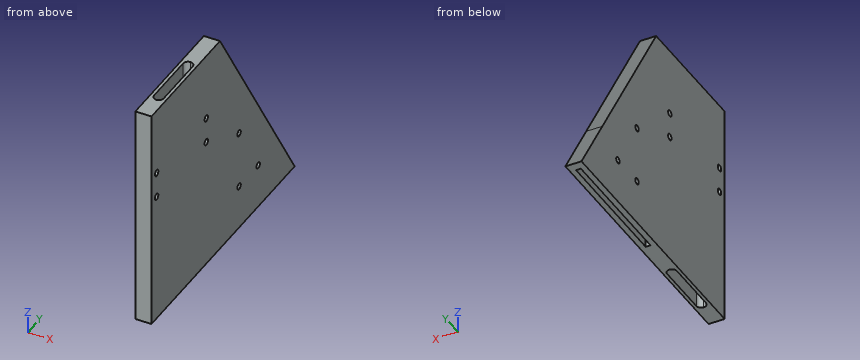
```python
from build123d import *

# Parameters (mm, degrees)
BOSS_EXTRUDE1_DEPTH   = 177.8
BOSS_EXTRUDE2_DEPTH   = 12.7
BOSS_EXTRUDE4_DEPTH   = 4.445
BOSS_EXTRUDE5_DEPTH   = 4.445
M6X1_0_TAPPED_HOLE1_D = 5
M6X1_0_TAPPED_HOLE2_D = 5


with BuildPart() as part:
    # Sketch1 → Boss-Extrude1 (new body)
    with BuildSketch(Plane.XY):
        with BuildLine():
            Line((0, 88.9), (0, 44.45))
            Line((0, 44.45), (2.54, 44.45))
            Line((2.54, 44.45), (2.54, 66.04))
            ThreePointArc((2.54, 66.04), (3.655923164, 68.734076836), (6.35, 69.85))
            ThreePointArc((6.35, 69.85), (9.044076836, 68.734076836), (10.16, 66.04))
            Line((10.16, 66.04), (10.16, 44.45))
            Line((10.16, 44.45), (12.7, 44.45))
            Line((12.7, 44.45), (12.7, 88.9))
            Line((12.7, 88.9), (0, 88.9))
        make_face()
        with BuildLine():
            Line((0, 44.45), (0, 0))
            Line((0, 0), (12.7, 0))
            Line((12.7, 0), (12.7, 44.45))
            Line((12.7, 44.45), (10.16, 44.45))
            Line((10.16, 44.45), (10.16, 22.86))
            ThreePointArc((10.16, 22.86), (9.044076836, 20.165923164), (6.35, 19.05))
            ThreePointArc((6.35, 19.05), (3.655923164, 20.165923164), (2.54, 22.86))
            Line((2.54, 22.86), (2.54, 44.45))
            Line((2.54, 44.45), (0, 44.45))
        make_face()
    extrude(amount=BOSS_EXTRUDE1_DEPTH)

    # Sketch5 → Boss-Extrude2 (add)
    with BuildSketch(Plane(origin=(0, 0, 0), x_dir=(0, 0, -1), z_dir=(1, 0, 0))):
        Polygon((-177.8, 101.6), (-177.8, 88.9), (0, 88.9), (0, 101.6), (-12.013513514, 101.6), (-165.786486486, 101.6), align=None)
        Polygon((-49.675142857, 181.378572199), (-177.8, 101.6), (-165.786486486, 101.6), (-88.904700233, 149.471422238), (-46.318714286, 175.988128132), align=None)
        Polygon((0, 212.309431825), (-49.675142857, 181.378572199), (-46.318714286, 175.988128132), (0, 204.82906481), align=None)
    extrude(amount=BOSS_EXTRUDE2_DEPTH)

    # Sketch6 → Boss-Extrude4 (add)
    with BuildSketch(Plane(origin=(12.7, 0, 0), x_dir=(0, 0, -1), z_dir=(1, 0, 0))):
        Polygon((-88.904700233, 149.471422238), (-165.786486486, 101.6), (-12.013513514, 101.6), (-3.356428571, 106.990444068), (-46.318714286, 175.988128132), align=None)
        Polygon((0, 204.82906481), (-46.318714286, 175.988128132), (-3.356428571, 106.990444068), (0, 109.080367015), align=None)
        Polygon((-12.013513514, 101.6), (0, 101.6), (-3.356428571, 106.990444068), align=None)
        Polygon((-3.356428571, 106.990444068), (0, 101.6), (0, 109.080367015), align=None)
    extrude(amount=-BOSS_EXTRUDE4_DEPTH)

    # Sketch5<6> → Boss-Extrude5 (add)
    with BuildSketch(Plane(origin=(0, 0, 0), x_dir=(0, 0, -1), z_dir=(1, 0, 0))):
        Polygon((-88.904700233, 149.471422238), (-165.786486486, 101.6), (-12.013513514, 101.6), (-3.356428571, 106.990444068), (-46.318714286, 175.988128132), align=None)
        Polygon((0, 204.82906481), (-46.318714286, 175.988128132), (-3.356428571, 106.990444068), (0, 109.080367015), align=None)
        Polygon((-12.013513514, 101.6), (0, 101.6), (-3.356428571, 106.990444068), align=None)
        Polygon((-3.356428571, 106.990444068), (0, 101.6), (0, 109.080367015), align=None)
    extrude(amount=BOSS_EXTRUDE5_DEPTH)

    # M6x1.0 Tapped Hole1 (through all)
    with Locations(Plane(origin=(12.7, 0, 0), x_dir=(0, 0, -1), z_dir=(1, 0, 0))):
        with Locations((-124.46, 7.62), (-104.14, 81.28), (-124.46, 81.28), (-104.14, 7.62)):
            Hole(M6X1_0_TAPPED_HOLE1_D / 2)

    # M6x1.0 Tapped Hole2 (through all)
    with Locations(Plane(origin=(0, 0, 0), x_dir=(0, 0, -1), z_dir=(-1, 0, 0))):
        with Locations((-35.287182484, -129.93571152), (-80.794502188, -129.93571152), (-35.287182484, -158.271423041)):
            Hole(M6X1_0_TAPPED_HOLE2_D / 2)


solid = part.part
```
Source: CAD feature listing. Evaluate the final solid. Frame: model axes, mm. Coordinates: 2 decimals unless noted, no trailing zeros. Loops run counter-clockwise (first coordinate to the right, second up) from the corner with the lowest first, then second, coordinate; pieces in that order, holes last. Notation, with made-up numbers: M -13,-31 L 39,-31 A30 cw 39,-9 Z; hole C -10,36 d11. An arc over 180 degrees is marked long. Use a Markdown table: item, result. Add a question column.
Q1. First-contact query: pin 1 (1.5 mm diameter, centred on x = 3.5, z = 105.5, fed in from +Y); pin 2 (1.9 mm diameter, centred on x = 6.5, z = 62, fed in from +Y); pin 3 (3 mm diameter, centred on x = 6, y = 186.5, fed in from -Z). Flat tips, straight axial feed; report the tip coordinate or a pass-through.
Q2. Section query B-B, the plane z = 104.14. Return loops of the section in (x, y) (3 decimals), and give its area (3 significant figures).
Q3. Section query C-C, the plane y = 7.62. Return loops of the section in (x, z).
Q4. Section query D-D, the plane z = 81. Return loops of the section in (x, y) (3 decimals).
Q5. Material intervals for L1, parallel to Y at x = 4.5, z = 57; L2, parallel to Y at x = 5.25, z = 44; L3, parallel to X at y = 132.5, z = 48.5 (3 decimals), sorted ascending.
Q6. Section query A-A, the plane y = 33. Return loops of the section in (x, z).
Result:
| question | item | result |
|---|---|---|
| 1 | pin 1 | stops at y = 147.09 |
| 1 | pin 2 | stops at y = 174.3 |
| 1 | pin 3 | stops at z = 27.03 |
| 2 | outline | M 0,0 L 12.7,0 L 12.7,5.12 L 0,5.12 Z; M 0,10.12 L 12.7,10.12 L 12.7,78.78 L 0,78.78 Z; M 0,83.78 L 12.7,83.78 L 12.7,147.465 L 0,147.465 Z; hole M 2.54,22.86 A3.81 ccw 10.16,22.86 L 10.16,66.04 A3.81 ccw 2.54,66.04 Z; hole M 4.445,101.6 L 8.255,101.6 L 8.255,139.985 L 4.445,139.985 Z |
| 2 | area | 1,220 mm2 |
| 3 | outline | M 0,0 L 12.7,0 L 12.7,101.64 L 0,101.64 Z; M 0,106.64 L 12.7,106.64 L 12.7,121.96 L 0,121.96 Z; M 0,126.96 L 12.7,126.96 L 12.7,177.8 L 0,177.8 Z |
| 4 | outline | M 0,0 L 12.7,0 L 12.7,127.444 L 8.255,127.444 L 8.255,101.6 L 4.445,101.6 L 4.445,127.444 L 0,127.444 Z; M 0,132.427 L 4.445,132.427 L 4.445,154.393 L 8.255,154.393 L 8.255,132.427 L 12.7,132.427 L 12.7,161.874 L 0,161.874 Z; hole M 2.54,22.86 A3.81 ccw 10.16,22.86 L 10.16,66.04 A3.81 ccw 2.54,66.04 Z |
| 5 | L1 | y = 0 to 19.53, 69.37 to 101.6, 169.34 to 176.82 |
| 5 | L2 | y = 0 to 19.21, 69.69 to 101.6, 177.43 to 184.91 |
| 5 | L3 | x = 0 to 4.445, 8.255 to 12.7 |
| 6 | outline | M 0,0 L 2.54,0 L 2.54,177.8 L 0,177.8 Z; M 10.16,0 L 12.7,0 L 12.7,177.8 L 10.16,177.8 Z |
